The listing builds one solid part. Answer for the finished solid, in the listing's coordinates (mm). A direction names the side the tool comes from. Coordinates: 2 decimals unless noted, no trailing zeros. Write each loop counter-clockwise with the first axis right and the second up, starting at its lowest first coordinate (ties: lowest second). Pieces come first, ordered by that corner, then holes. Notation, with made-up numbers: M -6.75,9.25 L 5.25,9.25 A12 ccw 5.25,26.25 Z; hole C 47,6 d3. An arc over 180 degrees is marked long. Put each result on its own line as item: value. Start each with the question number.
```python
from build123d import *

# Parameters (mm, degrees)
PAD_DEPTH       = 38.6
POCKET_DEPTH    = 16
POCKET001_DEPTH = 23
SKETCH003_W     = 39.120222
SKETCH003_H     = 14.384815
POCKET002_DEPTH = 23


with BuildPart() as part:
    # Sketch → Pad (new body)
    with BuildSketch(Plane.YZ):
        with BuildLine():
            Line((0, 0), (34.2, 0))
            Line((34.2, 0), (34.2, 6))
            ThreePointArc((34.2, 6), (33.32132, 8.12132), (31.2, 9))
            Line((31.2, 9), (3, 9))
            ThreePointArc((3, 9), (0.87868, 8.12132), (0, 6))
            Line((0, 6), (0, 0))
        make_face()
    extrude(amount=PAD_DEPTH)

    # Sketch001 (on Face7 of Pad) → Pocket (cut)
    with BuildSketch(Plane(origin=(0, 0, 0), x_dir=(0, 1, 0), z_dir=(-1, 0, 0))):
        Polygon((4, -3), (4, -1), (29, -1), (29, -2.704358), (33.2, -2.704358), (33.2, -5.204358), (29, -5.204358), (29, -7.5), (4, -7.5), (4, -5.5), (1, -5.5), (1, -3), align=None)
    extrude(amount=-POCKET_DEPTH, mode=Mode.SUBTRACT)

    # Sketch002 (on Face5 of Pocket) → Pocket001 (cut)
    with BuildSketch(Plane.YZ.offset(38.6)):
        with BuildLine():
            Line((1, 1), (33.2, 1))
            Line((33.2, 1), (33.2, 6))
            ThreePointArc((33.2, 6), (32.32132, 8.12132), (30.2, 9))
            Line((30.2, 9), (4, 9))
            ThreePointArc((4, 9), (1.87868, 8.12132), (1, 6))
            Line((1, 6), (1, 1))
        make_face()
    extrude(amount=-POCKET001_DEPTH, mode=Mode.SUBTRACT)

    # Sketch003 (on Face5 of Pocket001) → Pocket002 (cut)
    with BuildSketch(Plane.YZ.offset(38.6)):
        with Locations((18.894067, 10.192407)):
            Rectangle(SKETCH003_W, SKETCH003_H)
    extrude(amount=-POCKET002_DEPTH, mode=Mode.SUBTRACT)


solid = part.part
```
1) A cutting plane is placed at C-C on x = 15. Write down the section's boundary in (y, z).
2) A cutting plane is placed at B-B on z = 1.5. Write down the section's boundary in (x, y).
3) Determine the mould class of faces 1 (the face through (8, 17, 9)), 2 (the face through (8, 31, 2.704)), 3 (the face through (7.69, 0.9, 8.14)) for opening direction Y: +Y half, -Y half, draft (parallel to the pull), parting line (faces both ways), or undercut.
4) For faces 4 (the face through (19, 33.2, 2.6)), 5 (the face through (8, 17, 7.5)), 6 (the face through (27.3, 0.5, 3)), 7 (the face through (15.6, 2, 2)), 8 (the face through (15, 34.2, 2)), determine the directions among +Z, -Z, +X, -X, +Y, -Y from which every point of the face is accessible in a straight line to the end or side of a thin tool.
5) A cutting plane is placed at D-D on x = 35. Write down the section's boundary in (y, z), then the cut area to 3 significant figures.
6) Straight lines are drawn through the part: probe 1 along Z at (x, y) = (7, 3); probe 2 along Y at (x, z) = (4, 6); probe 3 along Z at (x, y) = (13.5, 21.5). For each, find the intervals that lie inside material, in ascending order.
7) Given pin 1 Ø1.5 at (x, y) = (31.5, 11.5) entering from +Z; pin 2 Ø1.6 at (x, z) = (6, 7) entering from +Y; pin 3 Ø1.1 at (x, y) = (28.5, 0.5) entering from +Z, each flat-ended and moving along its own axis, determine where each tip first touches the part or whether it passes through.
8) A cutting plane is placed at A-A on y = 17.5. Write down the section's boundary in (x, z), then the cut area to 3 significant figures.
Answers follow:
1. outline: M 0,0 L 34.2,0 L 34.2,6 A3 ccw 31.2,9 L 3,9 A3 ccw 0,6 Z; hole M 1,3 L 4,3 L 4,1 L 29,1 L 29,2.7 L 33.2,2.7 L 33.2,5.2 L 29,5.2 L 29,7.5 L 4,7.5 L 4,5.5 L 1,5.5 Z
2. outline: M 0,0 L 38.6,0 L 38.6,1 L 15.6,1 L 15.6,4 L 0,4 Z; M 0,29 L 15.6,29 L 15.6,33.2 L 38.6,33.2 L 38.6,34.2 L 0,34.2 Z
3. face 1: draft
3. face 2: undercut
3. face 3: -Y half
4. face 4: +X
4. face 5: +X, -X
4. face 6: +Z, +X, +Y, -Y
4. face 7: +Z, +X
4. face 8: +Z, -Z, +X, -X, +Y
5. outline: M 0,0 L 34.2,0 L 34.2,3 L 33.2,3 L 33.2,1 L 1,1 L 1,3 L 0,3 Z
5. area: 38.2 mm²
6. probe 1: z = 0 to 3, 5.5 to 9
6. probe 2: y = 0 to 4, 29 to 34.2
6. probe 3: z = 0 to 1, 7.5 to 9
7. pin 1: stops at z = 1
7. pin 2: stops at y = 34.19
7. pin 3: stops at z = 3
8. outline: M 0,0 L 38.6,0 L 38.6,1 L 0,1 Z; M 0,7.5 L 15.6,7.5 L 15.6,9 L 0,9 Z
8. area: 62.0 mm²
